```python
from build123d import *

# Parameters (mm, degrees)
SKETCH004_W   = 65
SKETCH004_H   = 30
SKETCH004_R   = 2.5
SKETCH004_W_2 = 12
SKETCH004_H_2 = 4.5
PAD003_DEPTH  = 2
FILLET004_R   = 1
FILLET005_R   = 1


with BuildPart() as part:
    # Sketch004 → Pad003 (new body)
    with BuildSketch(Plane.YZ):
        with Locations((0, 15)):
            Rectangle(SKETCH004_W, SKETCH004_H)
        with Locations((-14.5, 11)):
            Circle(SKETCH004_R, mode=Mode.SUBTRACT)
        with Locations((3.989801, 12.224792)):
            Rectangle(SKETCH004_W_2, SKETCH004_H_2, mode=Mode.SUBTRACT)
    extrude(amount=PAD003_DEPTH)

    # Fillet004
    fillet004_edges = [part.edges().sort_by_distance(p)[0] for p in [
        (2, 32.5, 15),
    ]]
    fillet(fillet004_edges, radius=FILLET004_R)

    # Fillet005
    fillet005_edges = [part.edges().sort_by_distance(p)[0] for p in [
        (2, -32.5, 15),
    ]]
    fillet(fillet005_edges, radius=FILLET005_R)


with BuildPart() as part_1:
    # Body003 placement: moved
    add(part.part.moved(Location((50.5, 0, 0))))


solid = part_1.part
```
The listing builds one solid part. Answer for the finished solid, in the listing's coordinates (mm). A direction names the side the tool comes from. Round coordinates to 2 decimals unless told otherwise and drop trailing zeros. Write each loop counter-clockwise with the first axis right and the second up, starting at its lowest first coordinate (ties: lowest second). Pieces come first, ordered by that corner, then holes. Notation, with made-up numbers: (-37.75, 65.5) -> (-33.75, 65.5) arc R25 ccw to (-33.75, 88.5) -> close; hole circle Ø11 at (46, 82). An arc over 180 degrees is marked (long way). Write item = value, one per line.
1) Section A-A on y = -16 is taken. Write down the section's boundary in (x, z), plus the area to 3 significant figures.
Check values:
outline = (50.5, 0) -> (52.5, 0) -> (52.5, 9) -> (50.5, 9) -> close; (50.5, 13) -> (52.5, 13) -> (52.5, 30) -> (50.5, 30) -> close
area = 52.0 mm²
2) Given pin 1 (3 mm diameter, centred on y = -14.5, z = 11, fed in from -X), flat-ended and moving along its own axis, determine where the tip first touches the part or whether it passes through.
Check values:
pin_1 = through
3) Which of the six approach directions +Z, -Z, +X, -X, +Y, -Y give full straight-line access (tool end or side, diameter ignored) to faces 4 (the flat face through (50.5, 0, 15)), 5 (the flat face through (51, 4, 14.475))?
Check values:
face_4 = +Z, -Z, -X, +Y, -Y
face_5 = +X, -X
4) For a pull along Z with two mould halves and no side action, classify faces 1 (the flat face through (51, 4, 9.975)), 2 (the flat face through (51, 0, 0)), 3 (the flat face through (52.5, 0, 15)) as released by +Z, released by -Z, zero draft, split by the parting line, or undercut.
Check values:
face_1 = undercut
face_2 = released by -Z
face_3 = zero draft
5) Section C-C on y = 1 is taken. Write down the section's boundary in (x, z).
Check values:
outline = (50.5, 0) -> (52.5, 0) -> (52.5, 9.97) -> (50.5, 9.97) -> close; (50.5, 14.47) -> (52.5, 14.47) -> (52.5, 30) -> (50.5, 30) -> close
6) Section B-B on z = 11 is taken. Write down the section's boundary in (x, y).
Check values:
outline = (50.5, -32.5) -> (51.5, -32.5) arc R1 ccw to (52.5, -31.5) -> (52.5, -17) -> (50.5, -17) -> close; (50.5, -12) -> (52.5, -12) -> (52.5, -2.01) -> (50.5, -2.01) -> close; (50.5, 9.99) -> (52.5, 9.99) -> (52.5, 31.5) arc R1 ccw to (51.5, 32.5) -> (50.5, 32.5) -> close
7) Straight lines are drawn through the part: line 1 along Z through (x, y) = (51.35, -14.5); line 2 along Z through (x, y) = (52.4, 0); line 3 along Y through (x, z) = (50.6, 12.75). For each, find the intervals that lie inside material, in ascending order. Write a range as [from, to].
Check values:
line_1 = [0, 8.5], [13.5, 30]
line_2 = [0, 9.97], [14.47, 30]
line_3 = [-32.5, -16.29], [-12.71, -2.01], [9.99, 32.5]
